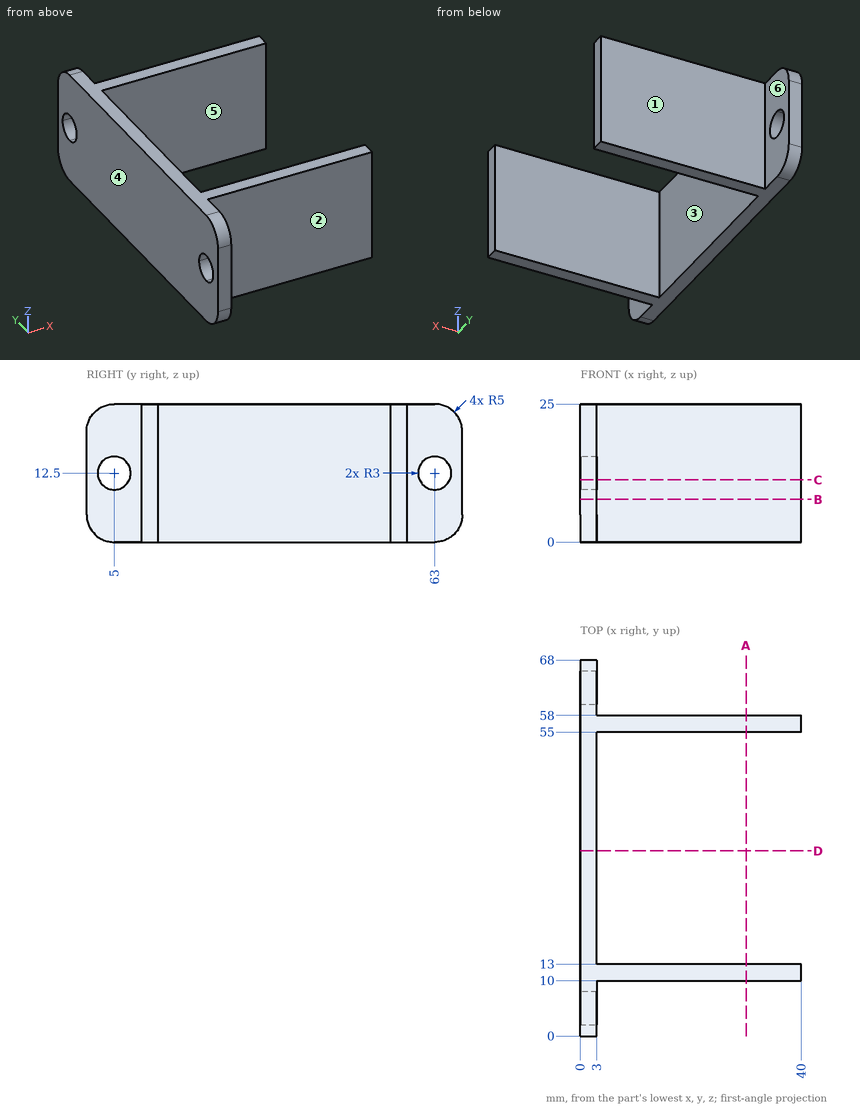
Can you work these out from the drawing? Everything is in mm from the part's minimum corner. A direction names the side the tool comes from. Round coordinates to 2 decimals unless told otherwise and drop trailing zeros. Loops run counter-clockwise (first coordinate to the right, second up) from the corner with the lowest first, then second, coordinate; pieces in that order, holes last. Notation, with made-up numbers: M 38,9.5 L 57,9.5 A27 cw 57,28.5 Z; hole C 17,88 d3. An arc over 180 degrees is marked long. Answer in a Markdown table with one row per item.
1. If we section it at D-D, the plane y = 33.5: Please give me the cut outline in (x, z), plus the area to 3 significant figures.
Established:
| item | result |
|---|---|
| outline | M 0,0 L 3,0 L 3,25 L 0,25 Z |
| area | 75.0 mm² |
2. If we section it at B-B, the plane z = 7.75: Please give me the cut outline in (x, y), plus the area to 3 significant figures.
Established:
| item | result |
|---|---|
| outline | M 0,0 L 3,0 L 3,10 L 40,10 L 40,13 L 3,13 L 3,55 L 40,55 L 40,58 L 3,58 L 3,68 L 0,68 Z |
| area | 426 mm² |
3. If we section it at C-C, the plane z = 11.25: Please give me the cut outline in (x, y).
Established:
| item | result |
|---|---|
| outline | M 0,0 L 3,0 L 3,2.27 L 0,2.27 Z; M 0,7.73 L 3,7.73 L 3,10 L 40,10 L 40,13 L 3,13 L 3,55 L 40,55 L 40,58 L 3,58 L 3,60.27 L 0,60.27 Z; M 0,65.73 L 3,65.73 L 3,68 L 0,68 Z |
4. On a 3-axis mill with a long thin cutter (end or side, diameter ignored), from which of +Z, -Z, +X, -X, +Y, -Y can I reach the whole of each face in a straight line? I mean the marked faces 5 and 6. Say none if no direction works.
Established:
| item | result |
|---|---|
| face 5 | +Z, -Z, +X |
| face 6 | +Z, -Z, +X, +Y |
5. If we section it at A-A, the plane x = 30: Please give me the cut outline in (y, z), plus the area to 3 significant figures.
Established:
| item | result |
|---|---|
| outline | M 10,0 L 13,0 L 13,25 L 10,25 Z; M 55,0 L 58,0 L 58,25 L 55,25 Z |
| area | 150 mm² |
6. Thinking about a two-plate mould opening in Y: for the marked faces 1, 2, 3 and 4, which applies, pulls with the +Y half, pulls with the -Y half, needs draft (parallel to the pull), parting line crosses it, or undercut?
Established:
| item | result |
|---|---|
| face 1 | pulls with the +Y half |
| face 2 | pulls with the -Y half |
| face 3 | undercut |
| face 4 | needs draft |
7. I'm going to push flat-ended pins straight in: pin 1 Ø12.5 at (x, z) = (19.5, 7.5) entering from -Y; pin 2 Ø4 at (y, z) = (32.5, 8) entering from +X; pin 3 Ø5 at (y, z) = (58, 19.5) entering from -X; pin 4 Ø12.5 at (x, z) = (22.5, 12.5) entering from +Y. Where does each tip first touch, or does it pass through?
Established:
| item | result |
|---|---|
| pin 1 | y = 10 |
| pin 2 | x = 3 |
| pin 3 | x = 0 |
| pin 4 | y = 58 |
8. Please list where these lines run through material, in increasing order: line 1 (Y direction, x = 22, z = 18.5); line 2 (X direction, y = 18, z = 6.75). Write a range as from..to.
Established:
| item | result |
|---|---|
| line 1 | 10..13, 55..58 |
| line 2 | 0..3 |
